Work out the finished part from the listing and answer in its coordinate system (mm). Round coordinates to 2 decimals unless told otherwise and drop trailing zeros. Write each loop counter-clockwise with the first axis right and the second up, starting at its lowest first coordinate (ties: lowest second). Pieces come first, ordered by that corner, then holes. Notation, with made-up numbers: (17.25, -22) - (51.25, -22) arc R22 ccw to (51.25, 11) - close; hole circle Ø7 at (18.5, 72.25). An arc over 180 degrees is marked (long way). Answer as a JSON object with one key per item and string values.
```python
from build123d import *

# Parameters (mm, degrees)
F0_R     = 30.1625
F1_DEPTH = 762
F3_D     = 42.8498


# Not quite as in the source:
# - a fillet or chamfer that OpenCascade refuses, or shapes differently, is made with other operations: its cross-section is extruded or revolved along the edge and cut away or added


with BuildPart() as f1:
    # F0 (on Front) → F1 (new body)
    with BuildSketch(Plane.XZ):
        Circle(F0_R)
    extrude(amount=F1_DEPTH)

    # F3 (through all)
    with Locations(Plane.XZ.offset(762)):
        with Locations((0, 0)):
            Hole(F3_D / 2)

    # F4: chamfer of 11.38682 on 2 edges, made by hand

    # F4_s1 → F4_t2 (revolve, cut)
    with BuildSketch(Plane.XY):
        Polygon((30.1625, -750.61318), (18.77568, -762), (30.1625, -762), align=None)
    revolve(axis=Axis((0, -762, 0), (0, -1, 0)), mode=Mode.SUBTRACT)

    # F4_s3 → F4_t4 (revolve, cut)
    with BuildSketch(Plane.XY):
        Polygon((30.1625, -11.38682), (18.77568, 0), (30.1625, 0), align=None)
    revolve(axis=Axis((0, 0, 0), (0, -1, 0)), mode=Mode.SUBTRACT)


solid = f1.part
```
Item 1: Consider line 1 along Z through (x, y) = (0, -227); line 2 along Z through (x, y) = (3.5, -109.5); line 3 along X through (y, z) = (-450, 8.5). Determine where each line is inside the solid, lowest interval first.
Results found:
{"line 1": "-30.16 to -21.42, 21.42 to 30.16", "line 2": "-29.96 to -21.14, 21.14 to 29.96", "line 3": "-28.94 to -19.67, 19.67 to 28.94"}
Item 2: A cutting plane is placed at A-A (z = 0). Write down the section's boundary in (x, y).
Results found:
{"outline": "(-30.16, -750.61) - (-21.42, -759.35) - (-21.42, -2.65) - (-30.16, -11.39) - close; (21.42, -759.35) - (30.16, -750.61) - (30.16, -11.39) - (21.42, -2.65) - close"}
Item 3: A cutting plane is placed at B-B (x = 0). Write down the section's boundary in (y, z), and give its area (3 significant figures).
Results found:
{"outline": "(-759.35, -21.42) - (-750.61, -30.16) - (-11.39, -30.16) - (-2.65, -21.42) - close; (-759.35, 21.42) - (-2.65, 21.42) - (-11.39, 30.16) - (-750.61, 30.16) - close", "area": "13,100 mm²"}
Item 4: Each of these flat-tipped pins is pushed along its axis until it touches: P1, Ø6, axis at y = -621, z = 0.5, coming from the +X side; P2, Ø10, axis at y = -130.5, z = -10, coming from the +X side; P3, Ø12, axis at y = -657, z = 12, coming from the -X side; P4, Ø3, axis at x = -21.5, z = -14, coming from the +Y side. Where does it stop, or does it pass through?
Results found:
{"P1": "x = 30.16", "P2": "x = 29.75", "P3": "x = -29.56", "P4": "y = -5.38"}
Item 5: A cutting plane is placed at C-C (y = -78). Write down the section's boundary in (x, z) (1 decimal).
Results found:
{"outline": "circle Ø60.3 at (0, 0); hole circle Ø42.8 at (0, 0)"}
Item 6: Determine the mould class of faces 1 (the cylindrical face through (2.789, -375.703, 21.243)), 2 (the conical face through (-17.34, -758.93, -13.29)) for opening direction Z: pulls with the +Z half, pulls with the -Z half, needs draft (parallel to the pull), parting line crosses it, or undercut.
Results found:
{"face 1": "undercut", "face 2": "parting line crosses it"}
